Geometry check sheet. Reference: the model listing, model coordinates, mm. Face numbers are marked on the shaded views. A direction names the side the tool comes from. Round coordinates to 2 decimals unless told otherwise and drop trailing zeros. Write each loop counter-clockwise with the first axis right and the second up, starting at its lowest first coordinate (ties: lowest second). Pieces come first, ordered by that corner, then holes. Notation, with made-up numbers: (31, 29.25) - (58, 29.25) arc R23 ccw to (58, 57.25) - close; hole circle Ø4 at (36, -26.75). An arc over 180 degrees is marked (long way). Return JSON: item names as keys, results as strings.
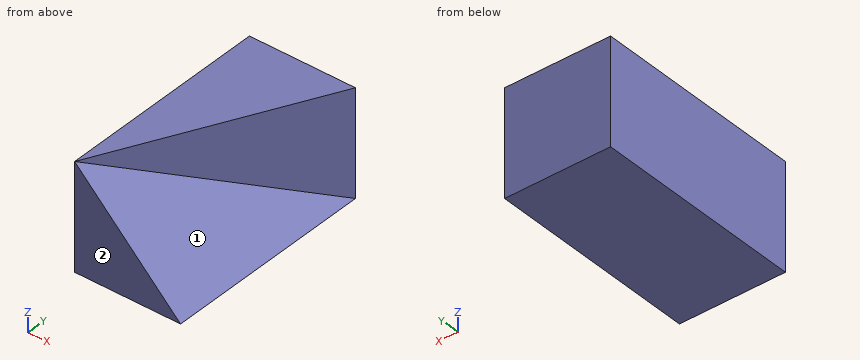
```python
from build123d import *

# Parameters (mm, degrees)
F1_DEPTH = 100
F3_DEPTH = 50


with BuildPart() as f1:
    # F0 (on Front) → F1 (new body)
    with BuildSketch(Plane.XZ):
        Polygon((0, 50), (0, 0), (50, 0), align=None)
    extrude(amount=-F1_DEPTH)

    # F2 (on face) → F3 (join, through all)
    with BuildSketch(Plane(origin=(0, 0, 0), x_dir=(1, 0, 0), z_dir=(0, 0, -1))):
        Polygon((50, -100), (0, 0), (0, -100), align=None)
    extrude(amount=-F3_DEPTH)


solid = f1.part
```
(1) Section check D-D, the plane x = 32. Enter the section's corners in (y, z), plus the area to 3 significant figures.
Response values:
{"outline": "(0, 0) - (100, 0) - (100, 50) - (64, 50) - (64, 18) - (0, 18) - close", "area": "2,950 mm^2"}
(2) Gauge pin test, flat ends, axial feed: pin 1 (2 mm diameter, centred on x = 42.5, y = 64.5, fed in from +Z); pin 2 (8 mm diameter, centred on y = 62, z = 34.5, fed in from +X); pin 3 (3 mm diameter, centred on x = 26.5, y = 17.5, fed in from +Z). Record the tip position at first contact, or that the pin passes through.
Response values:
{"pin 1": "stops at z = 8.5", "pin 2": "stops at x = 33", "pin 3": "stops at z = 25"}
(3) Access from +Z, -Z, +X, -X, +Y, -Y to the whole of each face (thin tool, end or side, straight path). Record for the marked faces 1 and 2.
Response values:
{"face 1": "+Z, +X, -Y", "face 2": "+Z, -Z, +X, -X, -Y"}
(4) Section check A-A, the plane y = 68. Enter the section's corners in (x, z).
Response values:
{"outline": "(0, 0) - (50, 0) - (34, 16) - (34, 50) - (0, 50) - close"}
(5) Section check B-B, the plane z = 14. Enter the section's corners in (x, y).
Response values:
{"outline": "(0, 0) - (36, 0) - (36, 72) - (50, 100) - (0, 100) - close"}
(6) Section check C-C, the plane x = 39. Enter the section's corners in (y, z), plus the area to 3 significant figures.
Response values:
{"outline": "(0, 0) - (100, 0) - (100, 50) - (78, 50) - (78, 11) - (0, 11) - close", "area": "1,960 mm^2"}
(7) Material ranges on line 1 along Y through (x, z) = (37.5, 27); line 2 along Y through (x, z) = (19, 42); line 3 along Z through (x, y) = (41.5, 54.5), recorded low to high. Write a range as [from, to].
Response values:
{"line 1": "y = [75, 100]", "line 2": "y = [38, 100]", "line 3": "z = [0, 8.5]"}
